Autodesk Inventor part; units mm, degrees
ref_plane "YZ Plane" through (0, 0, 0) normal (1, 0, 0) x (0, 1, 0)
ref_plane "XZ Plane" through (0, 0, 0) normal (0, 1, 0) x (-1, 0, 0)
ref_plane "XY Plane" through (0, 0, 0) normal (0, 0, 1) x (1, 0, 0)
sketch "Sketch1" plane through (0, 0, 0) normal (0, 1, 0) x (-1, 0, 0)
  line L0 (41.656, 38.862) -> (-59.944, 38.862)
  line L1 (-59.944, 38.862) -> (-59.944, -62.738)
  line L2 (-59.944, -62.738) -> (41.656, -62.738)
  line L3 (41.656, -62.738) -> (41.656, 38.862)
  circle A0 centre (-9.144, 19.812) radius 3.429
  circle A1 centre (-21.844, 19.812) radius 3.429
  circle A2 centre (-34.544, 19.812) radius 3.429
  circle A3 centre (-9.144, -43.688) radius 3.429
  circle A4 centre (-21.844, -43.688) radius 3.429
  circle A5 centre (-34.544, -43.688) radius 3.429
  point P0 (0, 0)
  point P1 (-9.144, 19.812)
  point P2 (-9.144, -43.688)
  point P3 (-9.144, -43.688)
  dimension "d0" = 101.6
  dimension "d1" = 101.6
  dimension "d3" = 6.858
  dimension "d4" = 12.7
  dimension "d5" = 12.7
  dimension "d6" = 25.4
  dimension "d8" = 19.05
  dimension "d9" = 19.05
  dimension "d10" = 6.858
  dimension "d11" = 12.7
  dimension "d12" = 12.7
extrude "Extrusion1" add sketch "Sketch1" along normal blind 1.5875
properties part number "Slider"
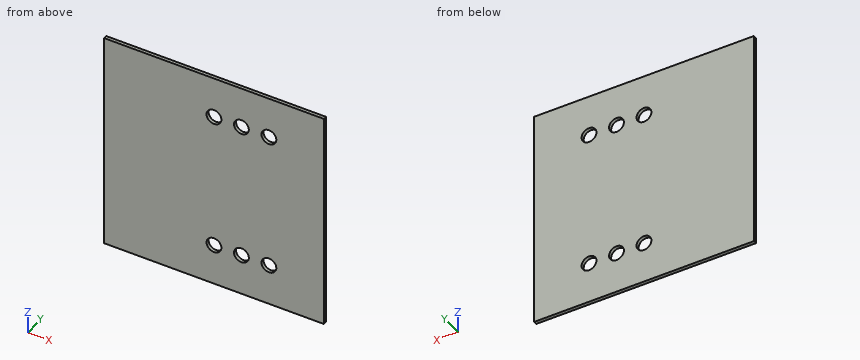
Source: CAD feature listing. Evaluate the final solid. Frame: model axes, mm. Coordinates: 2 decimals unless noted, no trailing zeros. Order: outer loops, then holes, each group sorted by start corner. A loop starts at its lowest first (then second) coordinate and runs counter-clockwise, first axis right, second up.
Item 1: Cut plane C-C (y = 0.7). Return loops of the section in (x, z) (3 decimals), plus the area to 3 significant figures.
Output values:
outline: (-41.656, -62.738) - (59.944, -62.738) - (59.944, 38.862) - (-41.656, 38.862) - close; hole circle Ø6.858 at (9.144, -43.688); hole circle Ø6.858 at (9.144, 19.812); hole circle Ø6.858 at (21.844, -43.688); hole circle Ø6.858 at (21.844, 19.812); hole circle Ø6.858 at (34.544, -43.688); hole circle Ø6.858 at (34.544, 19.812)
area: 10,100 mm2
Item 2: First-contact query: P1, Ø4, axis at x = 34.544, z = 19.812, coming from the +Y side. Flat tip, straight axial feed; report the tip coordinate or a pass-through.
Output values:
P1: passes through
Item 3: Material intervals for line 1 (X direction, y = 0.1, z = -43.5); line 2 (Z direction, x = 24.5, y = 1.4); line 3 (X direction, y = 1.4, z = -46.5), sorted ascending.
Output values:
line 1: x = -41.66 to 5.72, 12.57 to 18.42, 25.27 to 31.12, 37.97 to 59.94
line 2: z = -62.74 to -45.86, -41.52 to 17.64, 21.98 to 38.86
line 3: x = -41.66 to 7.18, 11.11 to 19.88, 23.81 to 32.58, 36.51 to 59.94
Item 4: Cut plane A-A (x = 20). Return loops of the section in (y, z).
Output values:
outline: (0, -62.74) - (1.59, -62.74) - (1.59, -46.58) - (0, -46.58) - close; (0, -40.8) - (1.59, -40.8) - (1.59, 16.92) - (0, 16.92) - close; (0, 22.7) - (1.59, 22.7) - (1.59, 38.86) - (0, 38.86) - close
Item 5: Cut plane B-B (z = 21). Return loops of the section in (x, y).
Output values:
outline: (-41.66, 0) - (5.93, 0) - (5.93, 1.59) - (-41.66, 1.59) - close; (12.36, 0) - (18.63, 0) - (18.63, 1.59) - (12.36, 1.59) - close; (25.06, 0) - (31.33, 0) - (31.33, 1.59) - (25.06, 1.59) - close; (37.76, 0) - (59.94, 0) - (59.94, 1.59) - (37.76, 1.59) - close
